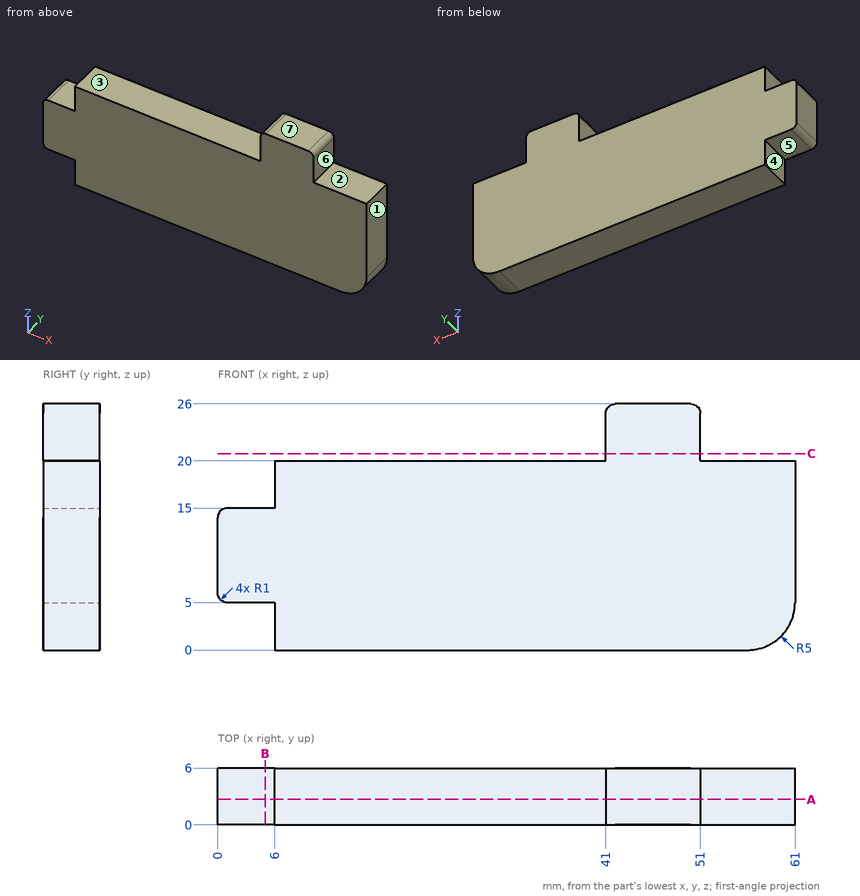
Could you check a few things on this drawing? It's one solid part, dimensions in mm from its lowest x, y, z. A direction names the side the tool comes from. Coordinates: 2 decimals unless noted, no trailing zeros. Loops run counter-clockwise (first coordinate to the right, second up) from the corner with the lowest first, then second, coordinate; pieces in that order, holes last. Notation, with made-up numbers: (56.25, 50.25) - (81.25, 50.25) arc R31 ccw to (81.25, 80.25) - close; hole circle Ø2 at (-34, 46). An arc over 180 degrees is marked (long way). Answer as a JSON object with one key per item and string values. Group by question number.
Item 1: If we section it at B-B (x = 5): List the corners of the cut face in (y, z) for me.
Item 2: If I drill on L1, parallel to Z at x = 26, y = 2.8; L2, parallel to X at y = 5.15, z = 22; L3, parallel to X at y = 2.7, z = 15.5, over which ranges is the centre line in solid material (lowest first)? Write a range as from..to.
Item 3: If we mould it in two halves opening along Z, with no side actions, what happens to the marked faces 5, 6 and 7? For each: released by +Z, released by -Z, zero draft, split by the parting line, or undercut.
Item 4: On a 3-axis mill with a long thin cutter (end or side, diameter ignored), from which of +Z, -Z, +X, -X, +Y, -Y can I reach the whole of each face in a straight line? I mean the marked faces 1, 2, 3 and 4. Say none if no direction works.
Item 5: If we section it at C-C (z = 20.75): List the corners of the cut face in (x, y) for me, plus the area to 3 significant figures.
Item 6: If we section it at A-A (y = 2.7): List the corners of the cut face in (x, z) for me.
Item 7: For pin 1 (2.5 mm diameter, centred on y = 3, z = 22.5, fed in from +X); pin 2 (1.8 mm diameter, centred on x = 21.5, y = 4, fed in from +Z), each with a flat end and sliding along its axis, tell me the tip position at first contact or that it passes through.
Returned:
{
 "1": {"outline": "(0, 5) - (6, 5) - (6, 15) - (0, 15) - close"},
 "2": {"L1": "z = 0..20", "L2": "x = 41..51", "L3": "x = 6..61"},
 "3": {"face 5": "released by -Z", "face 6": "zero draft", "face 7": "released by +Z"},
 "4": {"face 1": "+Z, -Z, +X, +Y, -Y", "face 2": "+Z, +X, +Y, -Y", "face 3": "+Z, -X, +Y, -Y", "face 4": "-Z, -X, +Y, -Y"},
 "5": {"outline": "(41, 0) - (51, 0) - (51, 6) - (41, 6) - close", "area": "60.0 mm²"},
 "6": {"outline": "(0, 6) arc R1 ccw to (1, 5) - (6, 5) - (6, 0) - (56, 0) arc R5 ccw to (61, 5) - (61, 20) - (51, 20) - (51, 25) arc R1 ccw to (50, 26) - (42, 26) arc R1 ccw to (41, 25) - (41, 20) - (6, 20) - (6, 15) - (1, 15) arc R1 ccw to (0, 14) - close"},
 "7": {"pin 1": "stops at x = 51", "pin 2": "stops at z = 20"}
}
